from build123d import *

# Parameters (mm, degrees)
F0_W     = 140
F0_H     = 50
F1_DEPTH = 110
F2_R     = 5
F3_T     = -3


with BuildPart() as f1:
    # F0 (on Top) → F1 (new body)
    with BuildSketch(Plane.XY):
        with Locations((-2.237636596, -25.9080916599)):
            Rectangle(F0_W, F0_H)
    extrude(amount=F1_DEPTH)

    # F2
    f2_edges = [f1.edges().sort_by_distance(p)[0] for p in [
        (-72.237637, -25.908092, 110),
        (67.762363, -25.908092, 110),
        (-2.237637, -50.908092, 0),
        (-2.237637, -0.908092, 0),
    ]]
    fillet(f2_edges, radius=F2_R)

    # F3
    f3_openings = [f1.faces().sort_by_distance(p)[0] for p in [
        (67.762363, -25.908092, 52.605233),
        (66.297897, -25.908092, 108.535534),
        (-2.237637, -25.908092, 110),
        (-70.773171, -25.908092, 108.535534),
        (-72.237637, -25.908092, 52.605233),
    ]]
    offset(amount=F3_T, openings=f3_openings)


solid = f1.part
Source: CAD feature listing. Evaluate the final solid. Frame: model axes, mm. A direction names the side the tool comes from. Round coordinates to 2 decimals unless told otherwise and drop trailing zeros. Loops run counter-clockwise (first coordinate to the right, second up) from the corner with the lowest first, then second, coordinate; pieces in that order, holes last.
Q1. Ray query, line 1 (Y direction, x = -53.5, z = 42.5); line 2 (Z direction, x = -57.5, y = -35.5); line 3 (Z direction, x = -65, y = -48). Return the intervals inside material, ascending.
Q2. Section B-B, the plane x = -60.5. Return loops of the section in (y, z).
Q3. Access query for faces 4 (the face through (-70.81, -49.39, 108.5)), 5 (the face through (-3, -26, 3)). Directions: +Z, -Z, +X, -X, +Y, -Y. A direction counts if a zero-diameter tool reaches every point of the face in a straight line with its end or side. Return the directions, or none.
Q4. Section A-A, the plane z = 43. Return loops of the section in (x, y).
Q5. First-contact query: P1, Ø12, axis at x = -8.5, y = -34, coming from the +Z side. Flat tip, straight axial feed; report the tip coordinate or a pass-through.
Q6. Section C-C, the plane y = -34. Return loops of the section in (x, z).
Q7. Mould query, pull axis Y, two halves, no side actions, for faces 1 (the face through (-72.238, -48.2, 44.5)), 2 (the face through (-1.258, -2.334, 1.504)), 3 (the face through (-3, -47.908, 57)). Classes: pulls with the +Y half, pulls with the -Y half, needs draft (parallel to the pull), parting line crosses it, or undercut.
Solutions:
1. line 1: y = -50.91 to -47.91, -3.91 to -0.91
1. line 2: z = 0 to 3
1. line 3: z = 0.46 to 110
2. outline: (-50.91, 5) arc R5 ccw to (-45.91, 0) - (-5.91, 0) arc R5 ccw to (-0.91, 5) - (-0.91, 110) - (-3.91, 110) - (-3.91, 5) arc R2 cw to (-5.91, 3) - (-45.91, 3) arc R2 cw to (-47.91, 5) - (-47.91, 110) - (-50.91, 110) - close
3. face 4: +Z, -X, +Y, -Y
3. face 5: +Z, +X, -X
4. outline: (-72.24, -50.91) - (67.76, -50.91) - (67.76, -47.91) - (-72.24, -47.91) - close; (-72.24, -3.91) - (67.76, -3.91) - (67.76, -0.91) - (-72.24, -0.91) - close
5. P1: stops at z = 3
6. outline: (-72.24, 0) - (67.76, 0) - (67.76, 3) - (-72.24, 3) - close
7. face 1: needs draft
7. face 2: pulls with the +Y half
7. face 3: undercut
